from build123d import *

# Parameters (mm, degrees)
F0_W     = 19.05
F0_H     = 19.05
F1_DEPTH = 63.5
F2_R     = 12.7
F3_DEPTH = 15.24
F4_R     = 9.525
F5_DEPTH = 25.4


with BuildPart() as f1:
    # F0 (on Front) → F1 (new body)
    with BuildSketch(Plane.XZ):
        with Locations((-16.331094, 12.57759)):
            Rectangle(F0_W, F0_H)
        with Locations((2.718906, 12.57759)):
            Rectangle(F0_W, F0_H)
        with Locations((-16.331094, -6.47241)):
            Rectangle(F0_W, F0_H)
        with Locations((2.718906, -6.47241)):
            Rectangle(F0_W, F0_H)
    extrude(amount=F1_DEPTH)

    # F2 (on face) → F3 (cut)
    with BuildSketch(Plane(origin=(0, 0, 0), x_dir=(-1, 0, 0), z_dir=(0, 1, 0))):
        with Locations((6.806094, 3.05259)):
            Circle(F2_R)
    extrude(amount=-F3_DEPTH, mode=Mode.SUBTRACT)

    # F4 (on face) → F5 (cut)
    with BuildSketch(Plane.XZ.offset(63.5)):
        with Locations((-5.737578, 3.05259)):
            Circle(F4_R)
    extrude(amount=-F5_DEPTH, mode=Mode.SUBTRACT)


solid = f1.part
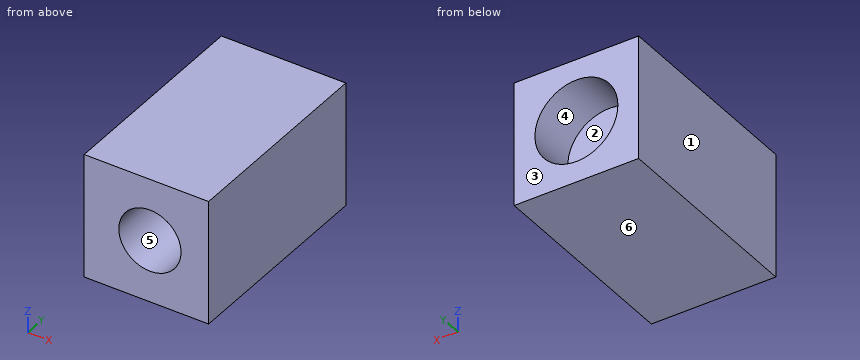
Read the model definition and answer for the solid it produces. Units are mm, in the model's axes. Face numbers are marked on the shaded views. A direction names the side the tool comes from. Round coordinates to 2 decimals unless told otherwise and drop trailing zeros. Write each loop counter-clockwise with the first axis right and the second up, starting at its lowest first coordinate (ties: lowest second). Pieces come first, ordered by that corner, then holes.
1. The part is cut by section B-B, the plane x = -11.5. Determine the outline of the cut face in (y, z), then the cut area to 3 significant figures.
2. Which of the six approach directions +Z, -Z, +X, -X, +Y, -Y give full straight-line access (tool end or side, diameter ignored) to the marked faces 4, 5 and 6?
3. Straight lines are drawn through the part: L1, parallel to Z at x = -9, y = -52; L2, parallel to Y at x = -9.5, z = 6.5; L3, parallel to Z at x = 0, y = -55. For each, find the intervals that lie inside material, in ascending order.
4. The part is cut by section A-A, the plane z = -3. Determine the outline of the cut face in (x, y), then the cut area to 3 significant figures.
5. Given pin 1 Ø5.5 at (x, z) = (-10, 2) entering from -Y, flat-ended and moving along its own axis, determine where the tip first touches the part or whether it passes through.
6. Determine the mould class of the marked faces 1, 2 and 3 for opening direction X: pulls with the +X half, pulls with the -X half, needs draft (parallel to the pull), parting line crosses it, or undercut.
7. The part is cut by section C-C, the plane y = -6. Determine the outline of the cut face in (x, z).
8. The part is cut by section D-D, the plane z = 13.5. Determine the outline of the cut face in (x, y), then the cut area to 3 significant figures.
Values:
1. outline: (-63.5, -16) - (0, -16) - (0, -8.75) - (-15.24, -8.75) - (-15.24, 14.85) - (0, 14.85) - (0, 22.1) - (-63.5, 22.1) - (-63.5, 10.64) - (-38.1, 10.64) - (-38.1, -4.53) - (-63.5, -4.53) - close
1. area: 1,670 mm2
2. face 4: +Y
2. face 5: -Y
2. face 6: -Z, +X, -X, +Y, -Y
3. L1: z = -16 to -5.9, 12 to 22.1
3. L2: y = -38.1 to -15.24
3. L3: z = -16 to -4.55, 10.66 to 22.1
4. outline: (-25.86, -63.5) - (-13.09, -63.5) - (-13.09, -38.1) - (1.62, -38.1) - (1.62, -63.5) - (12.24, -63.5) - (12.24, 0) - (4.36, 0) - (4.36, -15.24) - (-17.97, -15.24) - (-17.97, 0) - (-25.86, 0) - close
4. area: 1,710 mm2
5. pin 1: stops at y = -38.1
6. face 1: pulls with the -X half
6. face 2: undercut
6. face 3: needs draft
7. outline: (-25.86, -16) - (12.24, -16) - (12.24, 22.1) - (-25.86, 22.1) - close; hole circle Ø25.4 at (-6.81, 3.05)
8. outline: (-25.86, -63.5) - (12.24, -63.5) - (12.24, 0) - (0.41, 0) - (0.41, -15.24) - (-14.03, -15.24) - (-14.03, 0) - (-25.86, 0) - close
8. area: 2,200 mm2
